from build123d import *

# Parameters (mm, degrees)
SKETCH_1_R          = 45
EXTRUDE_1_DEPTH     = 10
SKETCH_2_R          = 2.75
CUT_EXTRUDE_1_DEPTH = 65.420493634
EXTRUDE_START       = -5
EXTRUDE_2_DEPTH     = 5
EXTRUDE_3_DEPTH     = 5
EXTRUDE_START_2     = 10
EXTRUDE_4_DEPTH     = 10
SKETCH_6_R          = 18.25
EXTRUDE_5_DEPTH     = 25
EXTRUDE_6_DEPTH     = 25
EXTRUDE_7_DEPTH     = 25
EXTRUDE_START_3     = 5
EXTRUDE_8_DEPTH     = 5
CHAMFER_1_SIZE      = 0.5
CHAMFER_2_SIZE      = 0.5
CHAMFER_3_SIZE      = 0.5
CHAMFER_4_SIZE      = 0.5
CHAMFER_5_SIZE      = 0.5
SKETCH_10_R         = 12.5
CUT_EXTRUDE_2_DEPTH = 194.971647413


with BuildPart() as part:
    # 草图1 → 凸台-拉伸1 (new body)
    with BuildSketch(Plane(origin=(0, 0, 0), x_dir=(0, 0, -1), z_dir=(1, 0, 0))):
        Circle(SKETCH_1_R)
    extrude(amount=EXTRUDE_1_DEPTH)

    # 草图2 → 切除-拉伸1 (cut, through all)
    with BuildSketch(Plane(origin=(10, 0, 0), x_dir=(0, 0, -1), z_dir=(1, 0, 0))):
        with Locations((0, 30)):
            Circle(SKETCH_2_R)
        with Locations((30, 0)):
            Circle(SKETCH_2_R)
        with Locations((0, -30)):
            Circle(SKETCH_2_R)
        with Locations((-30, 0)):
            Circle(SKETCH_2_R)
        with Locations((25.980762114, 15)):
            Circle(SKETCH_2_R)
        with Locations((15, 25.980762114)):
            Circle(SKETCH_2_R)
        with Locations(Location((-15, 25.980762114, 0), (0, 0, 180))):
            Circle(SKETCH_2_R)
        with Locations(Location((-25.980762114, 15, 0), (0, 0, 180))):
            Circle(SKETCH_2_R)
        with Locations((-25.980762114, -15)):
            Circle(SKETCH_2_R)
        with Locations((-15, -25.980762114)):
            Circle(SKETCH_2_R)
        with Locations(Location((15, -25.980762114, 0), (0, 0, 180))):
            Circle(SKETCH_2_R)
        with Locations(Location((25.980762114, -15, 0), (0, 0, 180))):
            Circle(SKETCH_2_R)
    extrude(amount=-CUT_EXTRUDE_1_DEPTH, mode=Mode.SUBTRACT)

    # 草图3 → 凸台-拉伸2 (add)
    with BuildSketch(Plane(origin=(10, 0, 0), x_dir=(0, 0, -1), z_dir=(1, 0, 0)).offset(EXTRUDE_START)):
        with BuildLine():
            ThreePointArc((45, 0), (0, -45), (-45, 0))
            Line((-45, 0), (-45, -80))
            Line((-45, -80), (45, -80))
            Line((45, -80), (45, 0))
        make_face()
    extrude(amount=EXTRUDE_2_DEPTH)

    # 草图4 → 凸台-拉伸3 (add)
    with BuildSketch(Plane.XZ.offset(80)):
        with BuildLine():
            Line((10, 45), (55, 45))
            ThreePointArc((55, 45), (100, 0), (55, -45))
            Line((55, -45), (10, -45))
            Line((10, -45), (10, 45))
        make_face()
    extrude(amount=-EXTRUDE_3_DEPTH)

    # 草图5 → 凸台-拉伸4 (add)
    with BuildSketch(Plane.XZ.offset(80).offset(EXTRUDE_START_2)):
        with BuildLine():
            Line((5, -45), (55, -45))
            ThreePointArc((55, -45), (100, 0), (55, 45))
            Line((55, 45), (5, 45))
            Line((5, 45), (5, -45))
        make_face()
    extrude(amount=-EXTRUDE_4_DEPTH)

    # 草图6 → 凸台-拉伸5 (add)
    with BuildSketch(Plane.XZ.offset(90)):
        with Locations(Location((55, 0, 0), (0, 0, 270))):
            Circle(SKETCH_6_R)
    extrude(amount=EXTRUDE_5_DEPTH)

    # 草图7 → 凸台-拉伸6 (add)
    with BuildSketch(Plane(origin=(0, 0, -45), x_dir=(-1, 0, 0), z_dir=(0, 0, -1))):
        Polygon((-40, -75), (-10, -50), (-10, -75), align=None)
    extrude(amount=-EXTRUDE_6_DEPTH)

    # 草图8 → 凸台-拉伸7 (add)
    with BuildSketch(Plane.XY.offset(45)):
        Polygon((10, -75), (40, -75), (10, -50), align=None)
    extrude(amount=-EXTRUDE_7_DEPTH)

    # 草图9 → 凸台-拉伸8 (add)
    with BuildSketch(Plane.ZY.offset(-5).offset(EXTRUDE_START_3)):
        with BuildLine():
            Line((-45, 0), (-45, -90))
            Line((-45, -90), (45, -90))
            Line((45, -90), (45, 0))
            ThreePointArc((45, 0), (0, -45), (-45, 0))
        make_face()
    extrude(amount=-EXTRUDE_8_DEPTH)

    # 倒角1
    chamfer_1_edges = [part.edges().sort_by_distance(p)[0] for p in [
        (55, -115, 18.25),
    ]]
    chamfer(chamfer_1_edges, length=CHAMFER_1_SIZE)

    # 倒角2
    chamfer_2_edges = [part.edges().sort_by_distance(p)[0] for p in [
        (10, -15, 28.730762114),
        (10, 15, 23.230762114),
        (10, 25.980762114, 12.25),
        (10, 25.980762114, -12.25),
        (10, 0, -27.25),
        (10, -30, 2.75),
        (10, 0, 32.75),
        (10, 15, -23.230762114),
        (10, -25.980762114, 17.75),
        (10, -25.980762114, -17.75),
        (10, -15, -28.730762114),
        (10, 30, 2.75),
    ]]
    chamfer(chamfer_2_edges, length=CHAMFER_2_SIZE)

    # 倒角3
    chamfer_3_edges = [part.edges().sort_by_distance(p)[0] for p in [
        (0, -45, -45),
        (0, -90, 0),
        (0, -45, 45),
        (0, 45, 0),
        (0, -15, 28.730762114),
        (0, 15, 23.230762114),
        (0, 25.980762114, 12.25),
        (0, 25.980762114, -12.25),
        (0, 0, -27.25),
        (0, -30, 2.75),
        (0, 0, 32.75),
        (0, 15, -23.230762114),
        (0, -25.980762114, 17.75),
        (0, -25.980762114, -17.75),
        (0, -15, -28.730762114),
        (0, 30, 2.75),
    ]]
    chamfer(chamfer_3_edges, length=CHAMFER_3_SIZE)

    # 倒角4
    chamfer_4_edges = [part.edges().sort_by_distance(p)[0] for p in [
        (10, -25, -45),
        (10, 45, 0),
        (10, -25, 45),
    ]]
    chamfer(chamfer_4_edges, length=CHAMFER_4_SIZE)

    # 倒角5
    chamfer_5_edges = [part.edges().sort_by_distance(p)[0] for p in [
        (25, -62.5, 20),
        (25, -62.5, -20),
        (24.75, -62.291666667, -45),
        (27.75, -90, -45),
        (27.75, -90, 45),
        (100, -90, 0),
        (100, -75, 0),
        (47.5, -75, -45),
        (47.5, -75, 45),
        (24.75, -62.291666667, 45),
    ]]
    chamfer(chamfer_5_edges, length=CHAMFER_5_SIZE)

    # 草图10 → 切除-拉伸2 (cut, through all)
    with BuildSketch(Plane.XZ.offset(115)):
        with Locations(Location((55, 0, 0), (0, 0, 270))):
            Circle(SKETCH_10_R)
    extrude(amount=-CUT_EXTRUDE_2_DEPTH, mode=Mode.SUBTRACT)


solid = part.part
Geometry check sheet. Reference: the model listing, model coordinates, mm. A direction names the side the tool comes from. Give positions to 0.01 mm unless a question says otherwise; leave off trailing zeros. Loops run counter-clockwise (first coordinate to the right, second up) from the corner with the lowest first, then second, coordinate; pieces in that order, holes last. Notation, with made-up numbers: (-15, -39) -> (-8, -39) arc R30 ccw to (-8, -12) -> close; hole circle Ø10 at (2.25, 10.5). An arc over 180 degrees is marked (long way). Answer in a Markdown table with one row per item. Add a question column.
1) Draft check along Y on faces 3 (the face through (0, -22, -1)), 4 (the face through (25.052, -62.864, 20.253)), 5 (the face through (5.063, -28.665, 15.596)). Enter one of: pulls with the +Y half, pulls with the -Y half, needs draft (parallel to the pull), parting line crosses it, or undercut.
2) Gauge pin test, flat ends, axial feed: P1, Ø9, axis at y = 15, z = -25.98, coming from the +X side; P2, Ø12, axis at y = -78.5, z = 6, coming from the +X side; P3, Ø3.5, axis at y = -15, z = -25.98, coming from the -X side; P4, Ø3, axis at x = 42, z = 11, coming from the +Y side. Record the tip position at first contact, or that the pin passes through.
3) Cross-section at A-A on y = -85. Record the boundary of the cut face in (x, z), and give its area (3 significant figures).
4) Cross-section at D-D on x = 29. Record the boundary of the cut face in (y, z), and give its area (3 significant figures).
5) Material ranges on probe 1 along Y at (x, z) = (3.25, 0); probe 2 along Y at (x, z) = (5.25, 15); probe 3 along Z at (x, y) = (4, -1.5), recorded low to high. Write a range as from..to.
6) Cross-section at C-C on z = 0. State how many separate pieces and enclosed holes the cut face has, and give its area (3 significant figures).
7) Cross-section at B-B on y = -15. Record the boundary of the cut face in (x, z).
8) Set-up check for faces 1 (the face through (0.135, 44.625, 0.982)), 2 (the face through (10, -14, 1)): record each of +Z, -Z, +X, -X, +Y, -Y from which the full face is reachable in a straight line by a thin tool's end or side.
Outcome:
| question | item | result |
|---|---|---|
| 1 | face 3 | needs draft |
| 1 | face 4 | pulls with the +Y half |
| 1 | face 5 | undercut |
| 2 | P1 | stops at x = 10 |
| 2 | P2 | stops at x = 100 |
| 2 | P3 | passes through |
| 2 | P4 | stops at y = -75 |
| 3 | outline | (0, -44.5) -> (0.5, -45) -> (55, -45) arc R45 ccw to (55, 45) -> (0.5, 45) -> (0, 44.5) -> close; hole circle Ø25 at (55, 0) |
| 3 | area | 7,640 mm^2 |
| 4 | outline | (-90, -44.5) -> (-89.5, -45) -> (-66.48, -45) -> (-65.83, -44.5) -> (-65.83, -20.5) -> (-66.48, -20) -> (-75, -20) -> (-75, 20) -> (-66.48, 20) -> (-65.83, 20.5) -> (-65.83, 44.5) -> (-66.48, 45) -> (-89.5, 45) -> (-90, 44.5) -> close |
| 4 | area | 1,810 mm^2 |
| 5 | probe 1 | y = -90..-32.75, -27.25..27.25, 32.75..45 |
| 5 | probe 2 | y = -90..-28.73, -23.23..23.23, 28.73..42.43 |
| 5 | probe 3 | z = -45..-32.3, -27.7..27.7, 32.3..45 |
| 6 | separate pieces | 4 |
| 6 | enclosed holes | 0 |
| 6 | area | 2,500 mm^2 |
| 7 | outline | (0, -44.5) -> (0.5, -45) -> (9.5, -45) -> (10, -44.5) -> (10, -29.23) -> (9.5, -28.73) -> (0.5, -28.73) -> (0, -29.23) -> close; (0, -22.73) -> (0.5, -23.23) -> (9.5, -23.23) -> (10, -22.73) -> (10, 22.73) -> (9.5, 23.23) -> (0.5, 23.23) -> (0, 22.73) -> close; (0, 29.23) -> (0.5, 28.73) -> (9.5, 28.73) -> (10, 29.23) -> (10, 44.5) -> (9.5, 45) -> (0.5, 45) -> (0, 44.5) -> close |
| 8 | face 1 | -X, +Y |
| 8 | face 2 | +X, +Y |
